from build123d import *

# Parameters (mm, degrees)
SKETCH1_R           = 5.926666667
BOSS_EXTRUDE1_DEPTH = 13.333333333
SKETCH2_R           = 6.426666667
BOSS_EXTRUDE2_DEPTH = 16.666666667
SKETCH3_R           = 6.426666667
BOSS_EXTRUDE3_DEPTH = 6.666666667
CHAMFER1_SIZE       = 2


with BuildPart() as part:
    # Sketch1 → Boss-Extrude1 (new body)
    with BuildSketch(Plane.XY):
        with Locations((137.157808662, 37.171292193)):
            Circle(SKETCH1_R)
    extrude(amount=BOSS_EXTRUDE1_DEPTH)

    # Sketch2 → Boss-Extrude2 (add)
    with BuildSketch(Plane.XY.offset(13.333333333)):
        with Locations((137.157808662, 37.171292193)):
            Circle(SKETCH2_R)
    extrude(amount=BOSS_EXTRUDE2_DEPTH)

    # Sketch3 → Boss-Extrude3 (add)
    with BuildSketch(Plane.XY.offset(30)):
        with Locations((137.157808662, 37.171292193)):
            Circle(SKETCH3_R)
    extrude(amount=BOSS_EXTRUDE3_DEPTH)

    # Chamfer1
    chamfer1_edges = [part.edges().sort_by_distance(p)[0] for p in [
        (130.731141995, 37.171292193, 36.666666667),
    ]]
    chamfer(chamfer1_edges, length=CHAMFER1_SIZE)


solid = part.part
Source: CAD feature listing. Evaluate the final solid. Frame: model axes, mm. A direction names the side the tool comes from. Give positions to 0.01 mm unless a question says otherwise; leave off trailing zeros. Write each loop counter-clockwise with the first axis right and the second up, starting at its lowest first coordinate (ties: lowest second). Pieces come first, ordered by that corner, then holes. Notation, with made-up numbers: M 36.25,-7 L 77.25,-7 A11 ccw 77.25,7 Z; hole C 22.25,19.5 d2. An arc over 180 degrees is marked long. Return JSON: item names as keys, results as strings. Group by question number.
1) Cut plane A-A, the plane z = 5. Output: boundary loops of the cut face in (x, y), plus the area to 3 significant figures.
2) Set-up query: faces 1 (the face through (137, 37, 36.667)), 2 (the face through (143, 35, 13.333)). Return all of +Z, -Z, +X, -X, +Y, -Y with unobstructed straight access to the full face (end or side cutting, diameter ignored); none if empty.
3) Material intervals for line 1 along X through (y, z) = (37.25, 7); line 2 along X through (y, z) = (37.5, 33); line 3 along Y through (x, z) = (133.5, 2.5), sorted ascending. Write a range as [from, to].
4) Cut plane B-B, the plane z = 27. Output: boundary loops of the cut face in (x, y).
5) Pin query (flat end, axial travel): P1, Ø6.5, axis at x = 137, y = 34, coming from the -Z side; P2, Ø2, axis at y = 41.5, z = 15.5, coming from the -X side; P3, Ø1, axis at x = 141.5, z = 7.5, coming from the -Y side; P4, Ø2, axis at x = 132.5, z = 21.5, coming from the -Y side. Return the tip coordinate at first contact, or that it passes through.
Recorded:
{
 "1": {"outline": "C 137.16,37.17 d11.85", "area": "110 mm²"},
 "2": {"face 1": "+Z, +X, -X, +Y, -Y", "face 2": "-Z"},
 "3": {"line 1": "x = [131.23, 143.08]", "line 2": "x = [130.74, 143.58]", "line 3": "y = [32.51, 41.83]"},
 "4": {"outline": "C 137.16,37.17 d12.85"},
 "5": {"P1": "stops at z = 0", "P2": "stops at x = 131.66", "P3": "stops at y = 32.66", "P4": "stops at y = 31.89"}
}
